Verification items for the finished model (mm, model axes). A direction names the side the tool comes from. Round coordinates to 2 decimals unless told otherwise and drop trailing zeros. Write each loop counter-clockwise with the first axis right and the second up, starting at its lowest first coordinate (ties: lowest second). Pieces come first, ordered by that corner, then holes. Notation, with made-up numbers: M 9,15.5 L 31,15.5 A15 ccw 31,32.5 Z; hole C -17,-32.5 d9. An arc over 180 degrees is marked long. One line per question, with ' | ' between items. Start each with the question number.
Q1. Cross-section at A-A (y = 35.5). Record the boundary of the cut face in (x, z).
Q2. Release check for a two-part mould opening along X. For faces 4 (the face through (133, 0, 3)), 5 (the face through (0, 24, 3)), 6 (the face through (128, 34, 4)) record: released by +X, released by -X, zero draft, split by the parting line, or undercut.
Q3. Tool access check on faces 1 (the face through (265, 15, 3)), 2 (the face through (137, 20, 2)), 3 (the face through (133, 24, 0)). Record the directions out of +Z, -Z, +X, -X, +Y, -Y that give a thin tool (end or side, any length) a straight path to the whole face; none if there is none.
Q4. Cross-section at C-C (x = 137.5). Record the boundary of the cut face in (y, z).
Q5. Gauge pin test, flat end, axial feed: pin 1 (2 mm diameter, centred on x = 188.5, y = 35, fed in from -Z). Record the tip position at first contact, or that the pin passes through.
Q6. Cross-section at B-B (z = 1.7). Record the boundary of the cut face in (x, y).
Q7. Thickness scan on line 1 along Y through (x, z) = (19.5, 2.05); line 2 along X through (y, z) = (19.5, 3.8); line 3 along Z through (x, y) = (116, 32). Record the ranges inside material, lowest first. Write a range as from..to.
Autodesk Fusion 360 part; units mm, degrees
sketch "Unsorted Smarties Top" plane through (0, 0, 0) normal (0, 0, 1) x (1, 0, 0)
  line L0 (0, 0) -> (270, 0)
  line L1 (270, 0) -> (270, 48)
  line L2 (270, 48) -> (0, 48)
  line L3 (0, 48) -> (0, 0)
  dimension "d1" = 270
  dimension "d2" = 48
extrude "Extrude1" add sketch "Unsorted Smarties Top" along normal blind 6
sketch "Sketch2" plane through (0, 0, 0) normal (0, 0, -1) x (1, 0, 0)
  line L0 (0, 0) -> (0, -48)
  line L1 (0, -48) -> (270, -48)
  line L2 (270, -48) -> (270, 0)
  line L3 (270, 0) -> (0, 0)
  line L4 (5, -10) -> (265, -10)
  line L5 (265, -10) -> (265, -20)
  line L6 (265, -20) -> (5, -20)
  line L7 (5, -20) -> (5, -10)
  line L8 (5, -29) -> (265, -29)
  line L9 (265, -29) -> (265, -39)
  line L10 (265, -39) -> (5, -39)
  line L11 (5, -39) -> (5, -29)
  dimension "d6" = 5
  dimension "d7" = 5
  dimension "d8" = 5
  dimension "d9" = 5
  dimension "d10" = 10
  dimension "d11" = 10
  dimension "d12" = 9
  dimension "d13" = 10
extrude "Extrude2" cut sketch "Sketch2" against normal blind 4 contours L4 L5 L6 L7 | L8 L9 L10 L11
sketch "Sketch3" plane through (0, 0, 4) normal (0, 0, -1) x (1, 0, 0)
  line L0 (5, -20) -> (265, -20)
  line L1 (265, -20) -> (265, -10)
  line L2 (265, -10) -> (5, -10)
  line L3 (5, -10) -> (5, -20)
  line L4 (265, -10) -> (255, -10)
  line L5 (255, -10) -> (255, -20)
  line L6 (255, -20) -> (265, -20)
  line L7 (265, -20) -> (265, -10)
  line L8 (265, -29) -> (255, -29)
  line L9 (255, -29) -> (255, -39)
  line L10 (255, -39) -> (265, -39)
  line L11 (265, -39) -> (265, -29)
extrude "Extrude3" cut sketch "Sketch3" against normal blind 2 contours L0 L1 L2 L4 L5 L6 L7 | L8 L9 L10 L11
equation "mdfThickness = 6 mm"
equation "d4 = mdfThickness"
Determined:
1) outline: M 0,0 L 5,0 L 5,4 L 255,4 L 255,6 L 0,6 Z; M 265,0 L 270,0 L 270,6 L 265,6 Z
2) face 4: zero draft | face 5: released by -X | face 6: undercut
3) face 1: +Z, -Z | face 2: -Z | face 3: -Z, +X, -X, +Y, -Y
4) outline: M 0,0 L 10,0 L 10,4 L 20,4 L 20,0 L 29,0 L 29,4 L 39,4 L 39,0 L 48,0 L 48,6 L 0,6 Z
5) pin 1: stops at z = 4
6) outline: M 0,0 L 270,0 L 270,48 L 0,48 Z; hole M 5,10 L 265,10 L 265,20 L 5,20 Z; hole M 5,29 L 265,29 L 265,39 L 5,39 Z
7) line 1: y = 0..10, 20..29, 39..48 | line 2: x = 0..5, 265..270 | line 3: z = 4..6
